Geometry check sheet. Reference: the model listing, model coordinates, mm. Round coordinates to 2 decimals unless told otherwise and drop trailing zeros. Order: outer loops, then holes, each group sorted by start corner. A loop starts at its lowest first (then second) coordinate and runs counter-clockwise, first axis right, second up. Notation, with made-up numbers: (76, -32) - (126, -32) arc R5 cw to (126, -28) - close; hole circle Ø5 at (-15, 4.25). An arc over 180 degrees is marked (long way). Use a Markdown table: item, result. Add a question column.
(1) Section check A-A on x = 0. Record the boundary of the cut face in (y, z), then the cut area to 3 significant figures.
(2) Section check B-B on z = 1.8. Record the boundary of the cut face in (x, y), then the cut area to 3 significant figures.
(3) Gauge pin test, flat end, axial feed: P1, Ø8, axis at x = 0, y = 30, coming from the +Z side. Record the tip position at first contact, or that the pin passes through.
(4) Thickness scan on line 1 along Y through (x, z) = (0, 0.6); line 2 along X through (y, z) = (8, 2.25); line 3 along Y through (x, z) = (1, 1.35). Record the ranges inside material, lowest first. Write a range as [from, to].
(5) Section check C-C on x = 14. Record the boundary of the cut face in (y, z).
(6) Section check D-D on x = 6.5. Record the boundary of the cut face in (y, z), then the cut area to 3 significant figures.
```python
from build123d import *

# Parameters (mm, degrees)
SALIENTE_EXTRUIR1_DEPTH           = 3
CORTAR_EXTRUIR1_REACH             = 52.71
CROQUIS3_R                        = 2.5
CROQUIS3_R_2                      = 5
CORTAR_EXTRUIR2_REACH             = 52.71
CROQUIS4_W                        = 8
CROQUIS4_H                        = 3
CORTAR_EXTRUIR2_DIRECTION_2_DEPTH = 51.709959574


with BuildPart() as part:
    # Croquis1 → Saliente-Extruir1 (new body)
    with BuildSketch(Plane.XY):
        with BuildLine():
            Line((-17.5, -30), (-17.5, 30))
            ThreePointArc((-17.5, 30), (0, 47.5), (17.5, 30))
            Line((17.5, 30), (17.5, -30))
            ThreePointArc((17.5, -30), (0, -47.5), (-17.5, -30))
        make_face()
    extrude(amount=SALIENTE_EXTRUIR1_DEPTH)

    # Croquis3 → Cortar-Extruir1 (cut, up to next)
    with BuildSketch(Plane.XY.offset(3), mode=Mode.PRIVATE) as cortar_extruir1_sk1:
        with Locations((0, 30)):
            Circle(CROQUIS3_R)
    cortar_extruir1_tool1 = extrude(cortar_extruir1_sk1.sketch, amount=-CORTAR_EXTRUIR1_REACH, mode=Mode.PRIVATE) & part.part
    # Croquis3 → Cortar-Extruir1 (cut, up to next)
    with BuildSketch(Plane.XY.offset(3), mode=Mode.PRIVATE) as cortar_extruir1_sk2:
        with Locations((0, -30)):
            Circle(CROQUIS3_R_2)
    cortar_extruir1_tool2 = extrude(cortar_extruir1_sk2.sketch, amount=-CORTAR_EXTRUIR1_REACH, mode=Mode.PRIVATE) & part.part
    add(cortar_extruir1_tool1.solids().sort_by_distance((0, 30, 3))[0], mode=Mode.SUBTRACT)
    add(cortar_extruir1_tool2.solids().sort_by_distance((0, -30, 3))[0], mode=Mode.SUBTRACT)

    # Croquis4 → Cortar-Extruir2 (cut, up to next)
    with BuildSketch(Plane.XY.offset(3), mode=Mode.PRIVATE) as cortar_extruir2_sk1:
        with Locations((0, 9.26)):
            Rectangle(CROQUIS4_W, CROQUIS4_H)
    cortar_extruir2_tool1 = extrude(cortar_extruir2_sk1.sketch, amount=-CORTAR_EXTRUIR2_REACH, mode=Mode.PRIVATE) & part.part
    add(cortar_extruir2_tool1.solids().sort_by_distance((0, 9.26, 3))[0], mode=Mode.SUBTRACT)

    # Croquis4 → Cortar-Extruir2 direction 2 (cut)
    with BuildSketch(Plane.XY.offset(3)):
        with Locations((0, 9.26)):
            Rectangle(CROQUIS4_W, CROQUIS4_H)
    extrude(amount=CORTAR_EXTRUIR2_DIRECTION_2_DEPTH, mode=Mode.SUBTRACT)


solid = part.part
```
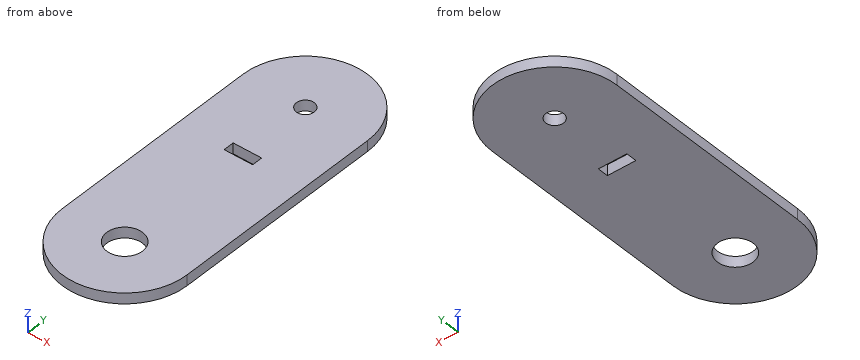
Check sheet entries:
| question | item | result |
|---|---|---|
| 1 | outline | (-47.5, 0) - (-35, 0) - (-35, 3) - (-47.5, 3) - close; (-25, 0) - (7.76, 0) - (7.76, 3) - (-25, 3) - close; (10.76, 0) - (27.5, 0) - (27.5, 3) - (10.76, 3) - close; (32.5, 0) - (47.5, 0) - (47.5, 3) - (32.5, 3) - close |
| 1 | area | 231 mm2 |
| 2 | outline | (-17.5, -30) arc R17.5 ccw to (17.5, -30) - (17.5, 30) arc R17.5 ccw to (-17.5, 30) - close; hole circle Ø10 at (0, -30); hole (-4, 7.76) - (4, 7.76) - (4, 10.76) - (-4, 10.76) - close; hole circle Ø5 at (0, 30) |
| 2 | area | 2,940 mm2 |
| 3 | P1 | stops at z = 3 |
| 4 | line 1 | y = [-47.5, -35], [-25, 7.76], [10.76, 27.5], [32.5, 47.5] |
| 4 | line 2 | x = [-17.5, -4], [4, 17.5] |
| 4 | line 3 | y = [-47.47, -34.9], [-25.1, 7.76], [10.76, 27.71], [32.29, 47.47] |
| 5 | outline | (-40.5, 0) - (40.5, 0) - (40.5, 3) - (-40.5, 3) - close |
| 6 | outline | (-46.25, 0) - (46.25, 0) - (46.25, 3) - (-46.25, 3) - close |
| 6 | area | 277 mm2 |
